Source: CAD feature listing. Evaluate the final solid. Frame: model axes, mm. A direction names the side the tool comes from. Coordinates: 2 decimals unless noted, no trailing zeros. Order: outer loops, then holes, each group sorted by start corner. A loop starts at its lowest first (then second) coordinate and runs counter-clockwise, first axis right, second up.
```python
from build123d import *

# Parameters (mm, degrees)
CYLINDER006_R          = 6
CYLINDER006_DEPTH      = 15
CYLINDER006_ROLL_ANGLE = 90
CYLINDER_R             = 10
CYLINDER_DEPTH         = 18
CYLINDER_ROLL_ANGLE    = 90


with BuildPart() as cylinder006:
    # Cylinder006 → Cylinder006 (new body)
    with BuildSketch(Plane.XY):
        Circle(CYLINDER006_R)
    extrude(amount=CYLINDER006_DEPTH)


with BuildPart() as cylinder006_1:
    # Cylinder006 roll: moved
    add(cylinder006.part.rotate(Axis((0, 0, 0), (1, 0, 0)), CYLINDER006_ROLL_ANGLE))


with BuildPart() as cylinder006_2:
    # Cylinder006 placement: moved
    add(cylinder006_1.part.moved(Location((450, 250, 50))))


with BuildPart() as obj1:
    # Cylinder → Cylinder (new body)
    with BuildSketch(Plane.XY):
        Circle(CYLINDER_R)
    extrude(amount=CYLINDER_DEPTH)


with BuildPart() as obj1_1:
    # Cylinder roll: moved
    add(obj1.part.rotate(Axis((0, 0, 0), (1, 0, 0)), CYLINDER_ROLL_ANGLE))


with BuildPart() as obj1_2:
    # Cylinder placement: moved
    add(obj1_1.part.moved(Location((450, 235, 50))))

    # Fusion: union Cylinder006
    add(cylinder006_2.part)


solid = obj1_2.part
```
Q1. Material intervals for line 1 along Y through (x, z) = (454, 58.5); line 2 along X through (y, z) = (240.5, 49.75); line 3 along Z through (x, y) = (455.75, 221), sorted ascending.
Solutions:
line 1: y = 217 to 235
line 2: x = 444.01 to 455.99
line 3: z = 41.82 to 58.18
Q2. Section query A-A on x = 450. Output: boundary loops of the cut face in (y, z).
Solutions:
outline: (217, 40) - (235, 40) - (235, 44) - (250, 44) - (250, 56) - (235, 56) - (235, 60) - (217, 60) - close
Q3. Section query D-D on z = 42.5. Output: boundary loops of the cut face in (x, y).
Solutions:
outline: (443.39, 217) - (456.61, 217) - (456.61, 235) - (443.39, 235) - close
Q4. Pin query (flat end, axial travel): P1, Ø3, axis at y = 227, z = 47.5, coming from the +X side; P2, Ø8, axis at x = 443, y = 232, coming from the -Z side; P3, Ø3, axis at y = 225.5, z = 57.5, coming from the +X side. Return the tip coordinate at first contact, or that it passes through.
Solutions:
P1: stops at x = 459.95
P2: stops at z = 40.46
P3: stops at x = 458
Q5. Set-up query: faces 1 (the flat face through (450, 217, 50)), 2 (the flat face through (450, 235, 43)). Return all of +Z, -Z, +X, -X, +Y, -Y with unobstructed straight access to the full face (end or side cutting, diameter ignored); none if empty.
Solutions:
face 1: +Z, -Z, +X, -X, -Y
face 2: +Y
Q6. Section query B-B on z = 50. Output: boundary loops of the cut face in (x, y), plus the area to 3 significant figures.
Solutions:
outline: (440, 217) - (460, 217) - (460, 235) - (456, 235) - (456, 250) - (444, 250) - (444, 235) - (440, 235) - close
area: 540 mm2
Q7. Section query C-C on y = 242. Output: boundary loops of the cut face in (x, z).
Solutions:
outline: circle Ø12 at (450, 50)
